Input: part model. Units: mm. Frame: model coordinates. Coordinates: 2 decimals unless noted, no trailing zeros. Loops run counter-clockwise (first coordinate to the right, second up) from the corner with the lowest first, then second, coordinate; pieces in that order, holes last.
(1) Contact query for flat-ended pins moving along their axis: P1, Ø2, axis at y = -26.5, z = 2, coming from the -X side; P2, Ø8, axis at x = 29.46, y = -9.51, coming from the -Z side; P3, Ø1.5, axis at y = -12, z = 0.5, coming from the -X side. Output: stop coordinate, or through.
(2) Section A-A, the plane z = 0.75. Return loops of the section in (x, y).
(3) Line query: L1, parallel to X at y = -9, z = 3.4; L2, parallel to Y at x = -28.5, z = 1.4; L3, parallel to Y at x = -60.5, z = 0.65. Output: solid intervals per line, ascending.
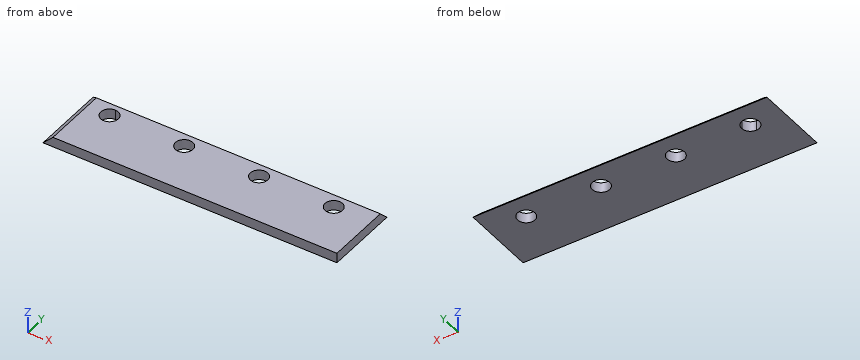
```python
from build123d import *

# Parameters (mm, degrees)
F0_R     = 3.5
F1_DEPTH = 4
F2_SIZE  = 3.99999


# Not quite as in the source:
# - a fillet or chamfer is up to 0.001 mm smaller than in the source, because OpenCascade refuses the exact size


with BuildPart() as f1:
    # F0 (on Top) → F1 (new body)
    with BuildSketch(Plane.XY):
        with BuildLine():
            Line((-60.536339879, 0), (-73.536339879, 0))
            Line((-73.536339879, 0), (-73.536339879, -4))
            Line((-73.536339879, -4), (-73.536339879, -30))
            Line((-73.536339879, -30), (-60.536339879, -30))
            Line((-60.536339879, -30), (-60.536339879, -13.0334984362))
            ThreePointArc((-60.536339879, -13.0334984362), (-64.036339879, -9.5334984362), (-60.536339879, -6.0334984362))
            Line((-60.536339879, -6.0334984362), (-60.536339879, 0))
        make_face()
        with BuildLine():
            Line((44.463660121, 0), (-60.536339879, 0))
            Line((-60.536339879, 0), (-60.536339879, -6.0334984362))
            ThreePointArc((-60.536339879, -6.0334984362), (-58.0614661449, -7.0586247021), (-57.036339879, -9.5334984362))
            ThreePointArc((-57.036339879, -9.5334984362), (-58.0614661449, -12.0083721704), (-60.536339879, -13.0334984362))
            Line((-60.536339879, -13.0334984362), (-60.536339879, -30))
            Line((-60.536339879, -30), (-52.7029968798, -30))
            Line((-52.7029968798, -30), (44.463660121, -30))
            Line((44.463660121, -30), (44.463660121, 0))
        make_face()
        with Locations((-30.536339879, -9.5774214715)):
            Circle(F0_R, mode=Mode.SUBTRACT)
        with Locations((-0.536339879, -9.52560734)):
            Circle(F0_R, mode=Mode.SUBTRACT)
        with Locations((29.463660121, -9.5145422965)):
            Circle(F0_R, mode=Mode.SUBTRACT)
    extrude(amount=F1_DEPTH)

    # F2 (size 4 in the source; OpenCascade refuses exactly that, so slightly less here)
    f2_edges = [f1.edges().sort_by_distance(p)[0] for p in [
        (-73.53634, -15, 4),
        (-14.53634, 0, 4),
    ]]
    chamfer(f2_edges, length=F2_SIZE)


solid = f1.part
```
Report:
1. P1: stops at x = -72.54
1. P2: stops at z = 0
1. P3: stops at x = -73.54
2. outline: (-72.79, -30) - (44.46, -30) - (44.46, -0.75) - (-72.79, -0.75) - close; hole circle Ø7 at (-60.54, -9.53); hole circle Ø7 at (-30.54, -9.58); hole circle Ø7 at (-0.54, -9.53); hole circle Ø7 at (29.46, -9.51)
3. L1: x = -70.14 to -64, -57.08 to -33.99, -27.08 to -4, 2.92 to 26, 32.93 to 44.46
3. L2: y = -30 to -12.42, -6.73 to -1.4
3. L3: y = -30 to -13.03, -6.03 to -0.65
